from build123d import *

# Parameters (mm, degrees)
SKETCH1_R           = 3.9497
BOSS_EXTRUDE1_DEPTH = 1.2954
SKETCH2_R           = 2.7305
SKETCH2_R_2         = 2.54
BOSS_EXTRUDE2_DEPTH = 6.1468
BOSS_EXTRUDE3_START = 3.8608
SKETCH3_W           = 1.0541
SKETCH3_H           = 0.968198064
SKETCH3_H_2         = 0.9906
BOSS_EXTRUDE3_DEPTH = 3.8608
SKETCH4_R           = 0.6223
BOSS_EXTRUDE4_DEPTH = 3.8608
SKETCH5_R           = 0.254
BOSS_EXTRUDE5_DEPTH = 6.35


with BuildPart() as part:
    # Sketch1 → Boss-Extrude1 (new body)
    with BuildSketch(Plane.XY):
        Circle(SKETCH1_R)
    extrude(amount=BOSS_EXTRUDE1_DEPTH)

    # Sketch2 → Boss-Extrude2 (add)
    with BuildSketch(Plane.XY.offset(1.2954)):
        Circle(SKETCH2_R)
        Circle(SKETCH2_R_2, mode=Mode.SUBTRACT)
    extrude(amount=BOSS_EXTRUDE2_DEPTH)

    # Sketch3 → Boss-Extrude3 (add)
    with BuildSketch(Plane(origin=(0, 0, 0), x_dir=(-1, 0, 0), z_dir=(0, 0, -1)).offset(BOSS_EXTRUDE3_START)):
        with Locations((2.52095, -0.011200968)):
            Rectangle(SKETCH3_W, SKETCH3_H)
        with Locations((-2.52095, 0)):
            Rectangle(SKETCH3_W, SKETCH3_H_2)
        with BuildLine():
            Line((-1.9939, -3.409471056), (-1.9939, -2.1971))
            Line((-1.9939, -2.1971), (-3.048, -2.1971))
            Line((-3.048, -2.1971), (-3.048, -2.511936721))
            ThreePointArc((-3.048, -2.511936721), (-2.560582136, -3.007249444), (-1.9939, -3.409471056))
        make_face()
        with BuildLine():
            Line((1.9939, -2.1971), (3.048, -2.1971))
            Line((3.048, -2.1971), (3.048, -2.511936721))
            ThreePointArc((3.048, -2.511936721), (2.560582136, -3.007249444), (1.9939, -3.409471056))
            Line((1.9939, -3.409471056), (1.9939, -2.1971))
        make_face()
    extrude(amount=-BOSS_EXTRUDE3_DEPTH)

    # Sketch4 → Boss-Extrude4 (add)
    with BuildSketch(Plane(origin=(0, 0, 0), x_dir=(-1, 0, 0), z_dir=(0, 0, -1))):
        with Locations(Location((0, 0, 0), (0, 0, 180))):
            Circle(SKETCH4_R)
    extrude(amount=BOSS_EXTRUDE4_DEPTH)

    # Sketch5 → Boss-Extrude5 (add)
    with BuildSketch(Plane.XY.offset(1.2954)):
        Circle(SKETCH5_R)
    extrude(amount=BOSS_EXTRUDE5_DEPTH)


solid = part.part
Geometry check sheet. Reference: the model listing, model coordinates, mm. A direction names the side the tool comes from. Round coordinates to 2 decimals unless told otherwise and drop trailing zeros. Write each loop counter-clockwise with the first axis right and the second up, starting at its lowest first coordinate (ties: lowest second). Pieces come first, ordered by that corner, then holes. Notation, with made-up numbers: (18.5, 89) -> (65.5, 89) arc R16 cw to (65.5, 107) -> close; hole circle Ø9 at (86.5, -32.5). An arc over 180 degrees is marked (long way). One line per item, written item: value. Start each with the question number.
(1) Cross-section at B-B, the plane x = 0. Record the cut outline in (y, z).
(2) Scan lines: line 1 (Y direction, x = 0, z = 5.5); line 2 (Z direction, x = -2, y = 1); line 3 (X direction, y = -0.5, z = 3.25). Record each from-to range of solid material in increasing order. Write a range as [from, to].
(3) Cross-section at C-C, the plane y = 0. Record the cut outline in (x, z).
(4) Cross-section at A-A, the plane z = -1. Record the cut outline in (x, y).
(5) Go/stop test with flat-tipped pins: pin 1 Ø0.6 at (y, z) = (-2.5, -2) entering from +X; pin 2 Ø0.8 at (y, z) = (0, -3) entering from -X; pin 3 Ø0.5 at (x, z) = (-2.5, -2.5) entering from +Y. Record where each tip stops, or that it passes through.
(6) Access from +Z, -Z, +X, -X, +Y, -Y to the whole of each face (thin tool, end or side, straight path). Record for faces 5 (the flat face through (-1.994, -3, -2)), 6 (the flat face through (-1, -3, 1.295)), 7 (the flat face through (2.5, -2.197, -2)).
(7) Cross-section at D-D, the plane z = 5.5. Record the cut outline in (x, y), and give its area (3 significant figures).
(8) Draft check along Y on faces 1 (the flat face through (-2.5, 0.473, -2)), 2 (the cylindrical face through (-0.33, 2.52, 4.33)), 3 (the cylindrical face through (2.604, 0.82, 4.326)), 4 (the flat face through (-2.5, 0, -3.861)). Enter one of: +Y half, -Y half, draft (parallel to the pull), parting line (faces both ways), or undercut.
Answer:
1. outline: (-3.95, 0) -> (-0.62, 0) -> (-0.62, -3.86) -> (0.62, -3.86) -> (0.62, 0) -> (3.95, 0) -> (3.95, 1.3) -> (2.73, 1.3) -> (2.73, 7.44) -> (2.54, 7.44) -> (2.54, 1.3) -> (0.25, 1.3) -> (0.25, 7.65) -> (-0.25, 7.65) -> (-0.25, 1.3) -> (-2.54, 1.3) -> (-2.54, 7.44) -> (-2.73, 7.44) -> (-2.73, 1.3) -> (-3.95, 1.3) -> close
2. line 1: [-2.73, -2.54], [-0.25, 0.25], [2.54, 2.73]
2. line 2: [0, 1.3]
2. line 3: [-2.68, -2.49], [2.49, 2.68]
3. outline: (-3.95, 0) -> (-3.05, 0) -> (-3.05, -3.86) -> (-1.99, -3.86) -> (-1.99, 0) -> (-0.62, 0) -> (-0.62, -3.86) -> (0.62, -3.86) -> (0.62, 0) -> (1.99, 0) -> (1.99, -3.86) -> (3.05, -3.86) -> (3.05, 0) -> (3.95, 0) -> (3.95, 1.3) -> (2.73, 1.3) -> (2.73, 7.44) -> (2.54, 7.44) -> (2.54, 1.3) -> (0.25, 1.3) -> (0.25, 7.65) -> (-0.25, 7.65) -> (-0.25, 1.3) -> (-2.54, 1.3) -> (-2.54, 7.44) -> (-2.73, 7.44) -> (-2.73, 1.3) -> (-3.95, 1.3) -> close
4. outline: (-3.05, -2.51) arc R3.95 ccw to (-1.99, -3.41) -> (-1.99, -2.2) -> (-3.05, -2.2) -> close; (-3.05, -0.5) -> (-1.99, -0.5) -> (-1.99, 0.47) -> (-3.05, 0.47) -> close; circle Ø1.24 at (0, 0); (1.99, -3.41) arc R3.95 ccw to (3.05, -2.51) -> (3.05, -2.2) -> (1.99, -2.2) -> close; (1.99, -0.5) -> (3.05, -0.5) -> (3.05, 0.5) -> (1.99, 0.5) -> close
5. pin 1: x = 3.05
5. pin 2: x = -3.05
5. pin 3: y = 0.47
6. face 5: -Z, +Y, -Y
6. face 6: +Z
6. face 7: -Z, +X, -X
7. outline: circle Ø5.46 at (0, 0); circle Ø0.51 at (0, 0); hole circle Ø5.08 at (0, 0)
7. area: 3.36 mm²
8. face 1: +Y half
8. face 2: undercut
8. face 3: parting line
8. face 4: draft
